The model under review builds one solid part; all positions refer to its coordinate system, in mm. Coordinates: 2 decimals unless noted, no trailing zeros. Loops run counter-clockwise (first coordinate to the right, second up) from the corner with the lowest first, then second, coordinate; pieces in that order, holes last. Notation, with made-up numbers: (8, 88) - (47, 88) arc R25 ccw to (47, 121) - close; hole circle Ø8 at (84, -21.5). An arc over 180 degrees is marked (long way). Answer in a Markdown table with one row per item. Add a question column.
(1) For line 1 along Y through (x, z) = (38.1, 1.45) (3 decimals); line 2 along X through (y, z) = (42, 1.7); line 3 along X through (y, z) = (14.5, 1), list the stretches that pass through material, from the lowest coordinate up.
(2) Mouldability with a two-part tool opening along Y and no side actions: class faces 1 (the cylindrical face through (0.91, 0.95, 1.16)), 2 (the flat face through (63, 27, 2.286)), 3 (the cylindrical face through (63.23, 39.21, 1.13)) as +Y half, -Y half, draft (parallel to the pull), parting line (faces both ways), or undercut.
(3) We need section A-A on y = 12.7. Write out the cut boundary in (x, z).
(4) For P1, Ø6.5, axis at x = 38.1, y = 12.7, coming from the -Z side, flat-tipped, find the tip position at first contact; note if it passes through.
(5) We need section D-D on x = 12. Write out the cut boundary in (y, z) (3 decimals).
(6) We need section C-C on z = 0.5. Give the number of separate pieces and of enclosed holes in the cut face, plus the area to 3 significant figures.
(7) We need section B-B on x = 63.5. Write out the cut boundary in (y, z) (3 decimals).
Autodesk Inventor part; units mm, degrees
ref_plane "YZ Plane" through (0, 0, 0) normal (1, 0, 0) x (0, 1, 0)
ref_plane "XZ Plane" through (0, 0, 0) normal (0, 1, 0) x (-1, 0, 0)
ref_plane "XY Plane" through (0, 0, 0) normal (0, 0, 1) x (1, 0, 0)
sketch "Sketch1" plane through (0, 0, 0) normal (0, 0, 1) x (1, 0, 0)
  line L0 (0, 0) -> (127, 0)
  line L1 (127, 0) -> (127, 53.975)
  line L2 (127, 53.975) -> (0, 53.975)
  line L3 (0, 53.975) -> (0, 0)
  line L4 (0, 53.975) -> (127, 53.975) construction
  line L5 (127, 53.975) -> (127, 26.9875) construction
  line L6 (127, 26.9875) -> (0, 26.9875) construction
  line L7 (0, 26.9875) -> (0, 53.975) construction
  circle A0 centre (114.3, 41.275) radius 2.0828
  circle A1 centre (88.9, 41.275) radius 2.0828
  circle A2 centre (63.5, 41.275) radius 2.0828
  line L8 (0, 26.9875) -> (127, 26.9875) construction
  circle A3 centre (114.3, 12.7) radius 2.0828
  circle A4 centre (88.9, 12.7) radius 2.0828
  circle A5 centre (63.5, 12.7) radius 2.0828
  circle A6 centre (38.1, 41.275) radius 2.0828
  circle A7 centre (12.7, 41.275) radius 2.0828
  circle A8 centre (38.1, 12.7) radius 2.0828
  circle A9 centre (12.7, 12.7) radius 2.0828
  dimension "d0" = 127
  dimension "d1" = 53.975
  dimension "d2" = 26.9875
  dimension "d3" = 4.1656
  dimension "d4" = 12.7
  dimension "d7" = 25.4
  dimension "d12" = 12.7
extrude "Plate1" add sketch "Sketch1" along normal blind 2.286
fillet "Fillet1" radius 3.175 4 edges at (127, 53.975, 1.143) (0, 53.975, 1.143) (127, 0, 1.143) (0, 0, 1.143)
equation "\"d2\" = 0.5 * d1"
equation "\"BendRadius\" = Thickness"
equation "\"BendReliefWidth\" = Thickness"
equation "\"BendReliefDepth\" = 0.5 * Thickness"
equation "\"CornerReliefSize\" = 4 * Thickness"
equation "\"MinimumRemnant\" = 2 * Thickness"
equation "\"TransitionRadius\" = BendRadius"
equation "\"JacobiRadiusSize\" = BendRadius"
equation "\"GapSize\" = Thickness"
equation "\"d13\" = BendRadius"
properties part number "Support for Connect Arm to Funnel  (Custom)" material "Aluminum 6061"
Outcome:
| question | item | result |
|---|---|---|
| 1 | line 1 | 0 to 10.617, 14.783 to 39.192, 43.358 to 53.975 |
| 1 | line 2 | 0 to 10.75, 14.65 to 36.15, 40.05 to 61.55, 65.45 to 86.95, 90.85 to 112.35, 116.25 to 127 |
| 1 | line 3 | 0 to 11.65, 13.75 to 37.05, 39.15 to 62.45, 64.55 to 87.85, 89.95 to 113.25, 115.35 to 127 |
| 2 | face 1 | -Y half |
| 2 | face 2 | draft |
| 2 | face 3 | undercut |
| 3 | outline | (0, 0) - (10.62, 0) - (10.62, 2.29) - (0, 2.29) - close; (14.78, 0) - (36.02, 0) - (36.02, 2.29) - (14.78, 2.29) - close; (40.18, 0) - (61.42, 0) - (61.42, 2.29) - (40.18, 2.29) - close; (65.58, 0) - (86.82, 0) - (86.82, 2.29) - (65.58, 2.29) - close; (90.98, 0) - (112.22, 0) - (112.22, 2.29) - (90.98, 2.29) - close; (116.38, 0) - (127, 0) - (127, 2.29) - (116.38, 2.29) - close |
| 4 | P1 | z = 0 |
| 5 | outline | (0, 0) - (10.738, 0) - (10.738, 2.286) - (0, 2.286) - close; (14.662, 0) - (39.313, 0) - (39.313, 2.286) - (14.662, 2.286) - close; (43.237, 0) - (53.975, 0) - (53.975, 2.286) - (43.237, 2.286) - close |
| 6 | separate pieces | 1 |
| 6 | enclosed holes | 10 |
| 6 | area | 6,710 mm² |
| 7 | outline | (0, 0) - (10.617, 0) - (10.617, 2.286) - (0, 2.286) - close; (14.783, 0) - (39.192, 0) - (39.192, 2.286) - (14.783, 2.286) - close; (43.358, 0) - (53.975, 0) - (53.975, 2.286) - (43.358, 2.286) - close |
